The drawing under review shows one solid part. Ordinate dimensions are in mm from its lowest x, y, z. A direction names the side the tool comes from. Give positions to 0.01 mm unless a question says otherwise; leave off trailing zeros. Loops run counter-clockwise (first coordinate to the right, second up) from the corner with the lowest first, then second, coordinate; pieces in that order, holes last.
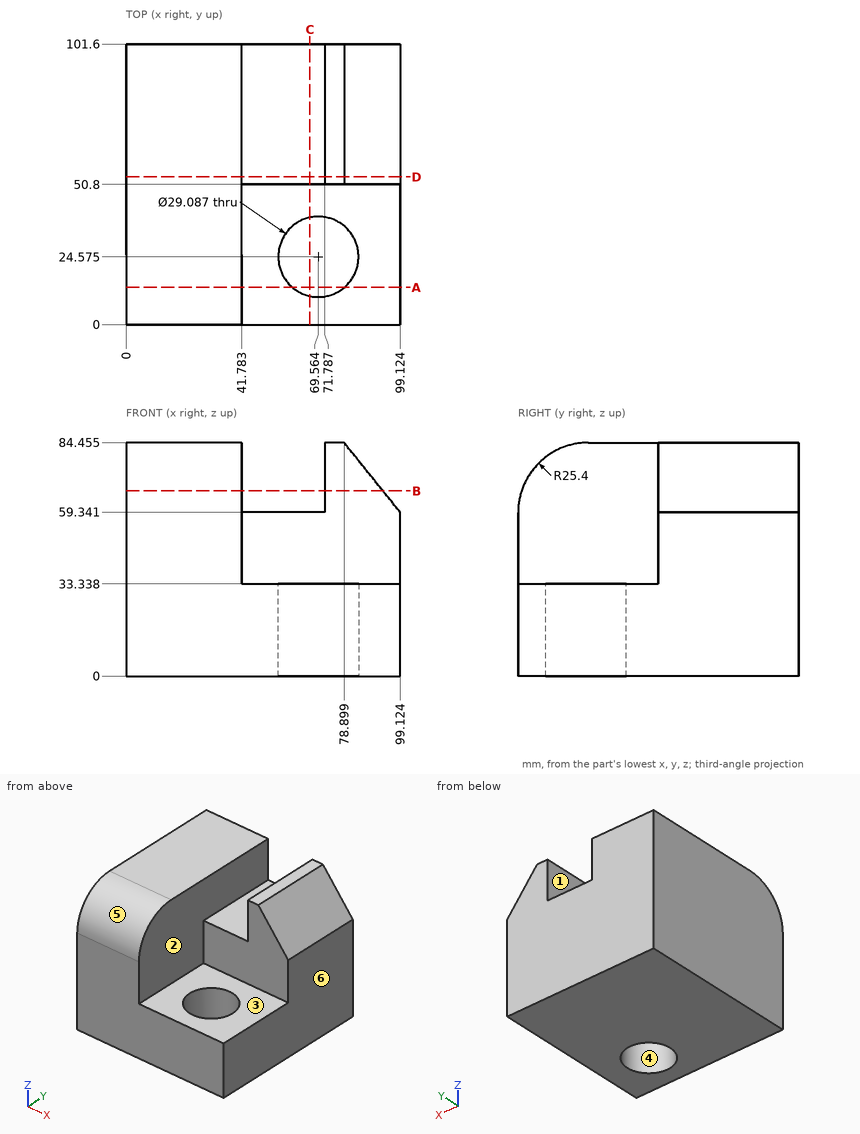
Item 1: Take a section at B-B on z = 67. Give the boundary of the cut face in (x, y) (1 decimal).
Answer:
outline: (0, 1.3) - (41.8, 1.3) - (41.8, 101.6) - (0, 101.6) - close; (71.8, 50.8) - (93, 50.8) - (93, 101.6) - (71.8, 101.6) - close
Item 2: Tool access review of the marked faces 1, 2 and 3: name each direction out of +Z, -Z, +X, -X, +Y, -Y from which nothing blocks a thin tool from reaching the whole face with its end or side.
Answer:
face 1: +Z, +Y, -Y
face 2: +Z, -Y
face 3: +Z, +X, -Y
Item 3: Clearance check with flat-ended pins moving along their axes: pin 1 Ø15.5 at (y, z) = (33.5, 62.5) entering from +X; pin 2 Ø12 at (x, z) = (65.5, 60.5) entering from -Y; pin 3 Ø3 at (x, y) = (54, 54) entering from +Z. State where each tip first meets the part, or that it passes through.
Answer:
pin 1: stops at x = 41.78
pin 2: stops at y = 50.8
pin 3: stops at z = 59.34
Item 4: The part is to be moulded in two halves that separate along Y. For the marked faces 4, 5 and 6, say which applies: released by +Y, released by -Y, zero draft, split by the parting line, or undercut.
Answer:
face 4: undercut
face 5: released by -Y
face 6: zero draft
Item 5: Take a section at D-D on y = 53.5. Give the boundary of the cut face in (x, z) (1 decimal), and give its area (3 significant figures).
Answer:
outline: (0, 0) - (99.1, 0) - (99.1, 59.3) - (78.9, 84.5) - (71.8, 84.5) - (71.8, 59.3) - (41.8, 59.3) - (41.8, 84.5) - (0, 84.5) - close
area: 7,360 mm2
Item 6: Take a section at A-A on y = 13.5. Give the boundary of the cut face in (x, z) (1 decimal), and give its area (3 significant figures).
Answer:
outline: (0, 0) - (60.1, 0) - (60.1, 33.3) - (41.8, 33.3) - (41.8, 81.5) - (0, 81.5) - close; (79, 0) - (99.1, 0) - (99.1, 33.3) - (79, 33.3) - close
area: 4,690 mm2
Item 7: For L1, parallel to X at y = 81, z = 60.5 (1 decimal); L2, parallel to Y at x = 63, z = 42; L3, parallel to X at y = 30, z = 30.5 (1 decimal), list the stretches that pass through material, from the lowest coordinate up.
Answer:
L1: x = 0 to 41.8, 71.8 to 98.2
L2: y = 50.8 to 101.6
L3: x = 0 to 56.1, 83.1 to 99.1
Item 8: Take a section at C-C on x = 66.5. Give the boundary of the cut face in (y, z).
Answer:
outline: (0, 0) - (10.36, 0) - (10.36, 33.34) - (0, 33.34) - close; (38.79, 0) - (101.6, 0) - (101.6, 59.34) - (50.8, 59.34) - (50.8, 33.34) - (38.79, 33.34) - close
